For this review, use the dimensioned drawing (mm, ordinates from the lowest corner) and the shaded views. Coordinates: 2 decimals unless noted, no trailing zeros. Write each loop counter-clockwise with the first axis right and the second up, starting at its lowest first coordinate (ties: lowest second). Pieces come first, ordered by that corner, then holes.
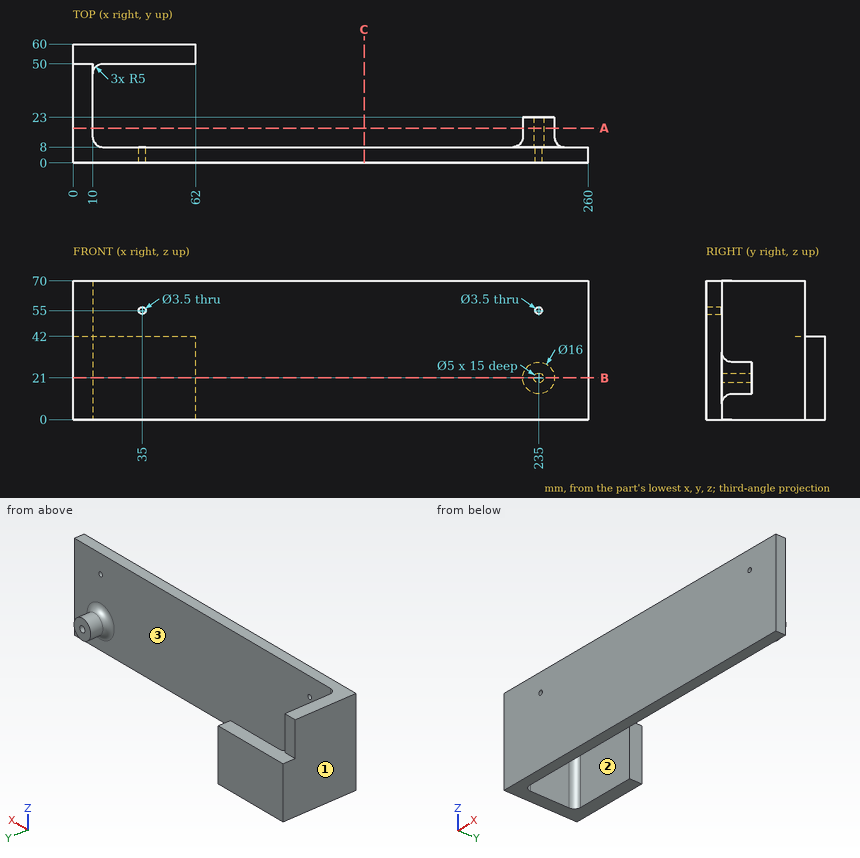
Item 1: Take a section at C-C, the plane x = 147. Write out the cut boundary in (y, z), plus the area to 3 significant figures.
Solved:
outline: (0, 0) - (8, 0) - (8, 70) - (0, 70) - close
area: 560 mm2
Item 2: For pin 1 (12 mm diameter, centred on x = 151, z = 31, fed in from +Y); pin 2 (11 mm diameter, centred on y = 23.5, z = 21, fed in from +X); pin 3 (13 mm diameter, centred on x = 238, z = 23.5, fed in from +Y), all flat-tipped, find the tip position at first contact; note any pin that passes through.
Solved:
pin 1: stops at y = 8
pin 2: stops at x = 243
pin 3: stops at y = 23
Item 3: Mouldability with a two-part tool opening along X and no side actions: class the marked faces 1, 2 and 3 as pulls with the +X half, pulls with the -X half, needs draft (parallel to the pull), parting line crosses it, or undercut.
Solved:
face 1: pulls with the -X half
face 2: needs draft
face 3: undercut
Item 4: To check wall thickness, follow line 1 along X through (y, z) = (5.5, 55); line 2 along X through (y, z) = (16.5, 21); line 3 along Y through (x, z) = (34, 39). State the ranges of each line that lie inside material, in increasing order.
Solved:
line 1: x = 0 to 33.25, 36.75 to 233.25, 236.75 to 260
line 2: x = 0 to 10, 227 to 232.5, 237.5 to 243
line 3: y = 0 to 8, 50 to 60
Item 5: Take a section at B-B, the plane z = 21. Write out the cut boundary in (x, y).
Solved:
outline: (0, 0) - (260, 0) - (260, 8) - (248, 8) arc R5 cw to (243, 13) - (243, 23) - (237.5, 23) - (237.5, 8) - (232.5, 8) - (232.5, 23) - (227, 23) - (227, 13) arc R5 cw to (222, 8) - (15, 8) arc R5 cw to (10, 13) - (10, 45) arc R5 cw to (15, 50) - (62, 50) - (62, 60) - (0, 60) - close
Item 6: Take a section at A-A, the plane y = 17.5. Write out the cut boundary in (x, z), plus the area to 3 significant figures.
Solved:
outline: (0, 0) - (10, 0) - (10, 70) - (0, 70) - close; circle Ø16 at (235, 21); hole circle Ø5 at (235, 21)
area: 881 mm2
